from build123d import *

# Parameters (mm, degrees)
CROQUIS1_R              = 1.5
CROQUIS1_W              = 15
CROQUIS1_H              = 15
SALIENTE_EXTRUIR1_DEPTH = 1
CROQUIS3_W              = 5
CROQUIS3_H              = 4.949226591
CROQUIS3_H_2            = 5
CORTAR_EXTRUIR2_DEPTH   = 10


with BuildPart() as part:
    # Croquis1 → Saliente-Extruir1 (new body)
    with BuildSketch(Plane(origin=(0, 0, 0), x_dir=(1, 0, 0), z_dir=(0, 1, 0))):
        with BuildLine():
            ThreePointArc((-15, -14.898453182), (-14.949747468, -14.949747468), (-14.898453182, -15))
            Line((-14.898453182, -15), (30, -15))
            Line((30, -15), (30, 30))
            Line((30, 30), (-15, 30))
            Line((-15, 30), (-15, -14.898453182))
        make_face()
        with Locations(Location((0.5, -10, 0), (0, 0, 270))):
            Circle(CROQUIS1_R, mode=Mode.SUBTRACT)
        with Locations(Location((-10.5, -3.75, 0), (0, 0, 270))):
            Circle(CROQUIS1_R, mode=Mode.SUBTRACT)
        with Locations(Location((14.5, -10, 0), (0, 0, 270))):
            Circle(CROQUIS1_R, mode=Mode.SUBTRACT)
        with Locations(Location((25.5, -3.75, 0), (0, 0, 270))):
            Circle(CROQUIS1_R, mode=Mode.SUBTRACT)
        with Locations(Location((-10.5, 18.75, 0), (0, 0, 270))):
            Circle(CROQUIS1_R, mode=Mode.SUBTRACT)
        with Locations(Location((0.5, 25, 0), (0, 0, 270))):
            Circle(CROQUIS1_R, mode=Mode.SUBTRACT)
        with Locations((7.5, 7.5)):
            Rectangle(CROQUIS1_W, CROQUIS1_H, mode=Mode.SUBTRACT)
        with Locations(Location((14.5, 25, 0), (0, 0, 270))):
            Circle(CROQUIS1_R, mode=Mode.SUBTRACT)
        with Locations(Location((25.5, 18.75, 0), (0, 0, 270))):
            Circle(CROQUIS1_R, mode=Mode.SUBTRACT)
    extrude(amount=SALIENTE_EXTRUIR1_DEPTH)

    # Croquis3 → Cortar-Extruir2 (cut)
    with BuildSketch(Plane(origin=(0, 1, 0), x_dir=(1, 0, 0), z_dir=(0, 1, 0))):
        with Locations((7.5, 27.525386705)):
            Rectangle(CROQUIS3_W, CROQUIS3_H)
        with Locations((7.5, -12.5)):
            Rectangle(CROQUIS3_W, CROQUIS3_H_2)
    extrude(amount=-CORTAR_EXTRUIR2_DEPTH, mode=Mode.SUBTRACT)


solid = part.part
Design review of the part built by this model. Coordinates are the model's own, in mm. A direction names the side the tool comes from. Give positions to 0.01 mm unless a question says otherwise; leave off trailing zeros. Order: outer loops, then holes, each group sorted by start corner. A loop starts at its lowest first (then second) coordinate and runs counter-clockwise, first axis right, second up. Notation, with made-up numbers: (69, 88) - (84, 88) arc R6 cw to (84, 98) - close; hole circle Ø4 at (85.5, 38). An arc over 180 degrees is marked (long way). Write item = value, one per line. Start each with the question number.
Q1. Clearance check with flat-ended pins moving along their axes: pin 1 Ø1.8 at (x, z) = (0.5, -25) entering from -Y; pin 2 Ø0.5 at (x, y) = (6.5, 0.5) entering from +Z; pin 3 Ø4 at (x, z) = (0.5, 10) entering from +Y; pin 4 Ø0.5 at (x, y) = (8.5, 0.5) entering from -Z. State where each tip first meets the part, or that it passes through.
Q2. Mouldability with a two-part tool opening along X and no side actions: class faces 5 (the face through (7.5, 0.5, -25.051)), 6 (the face through (30, 0.5, -7.2)), 7 (the face through (-4.9, 0.5, -30)) as released by +X, released by -X, zero draft, split by the parting line, or undercut.
Q3. Tool access review of faces 1 (the face through (7, 0, -18)), 2 (the face through (10, 0.5, -27.5)), 3 (the face through (10, 0.5, 12.5)), 4 (the face through (15, 0.5, -7.4)): name each direction out of +Z, -Z, +X, -X, +Y, -Y from which nothing blocks a thin tool from reaching the whole face with its end or side.
Q4. We need section A-A on z = -18.75. State the section outline as (x, y) points.
Q5. We need section B-B on y = 0.6. State how many separate pieces and enclosed holes the cut face has, plus the area to 3 significant figures.
Q6. We need section C-C on z = 3.5. State the section outline as (x, y) points.
Q7. To check wall thickness, follow L1, parallel to X at y = 0.5, z = 3.75; L2, parallel to X at y = 0.65, z = -25; L3, parallel to X at y = 0.5, z = -13. State the ranges of each line that lie inside material, in increasing order. Write a range as from..to.
Working result:
q1.pin_1 = through
q1.pin_2 = 10
q1.pin_3 = 1
q1.pin_4 = -25.05
q2.face_5 = undercut
q2.face_6 = released by +X
q2.face_7 = zero draft
q3.face_1 = +Z, -Z, +X, -X, -Y
q3.face_2 = -Z, +Y, -Y
q3.face_3 = +Z, +Y, -Y
q3.face_4 = +Y, -Y
q4.outline = (-15, 0) - (-12, 0) - (-12, 1) - (-15, 1) - close; (-9, 0) - (24, 0) - (24, 1) - (-9, 1) - close; (27, 0) - (30, 0) - (30, 1) - (27, 1) - close
q5.separate_pieces = 1
q5.enclosed_holes = 9
q5.area = 1,690 mm²
q6.outline = (-15, 0) - (-11.98, 0) - (-11.98, 1) - (-15, 1) - close; (-9.02, 0) - (24.02, 0) - (24.02, 1) - (-9.02, 1) - close; (26.98, 0) - (30, 0) - (30, 1) - (26.98, 1) - close
q7.L1 = -15..-12, -9..24, 27..30
q7.L2 = -15..-1, 2..13, 16..30
q7.L3 = -15..0, 15..30
